Could you check a few things on this model? Use its own coordinates, in mm. A direction names the side the tool comes from. Coordinates: 2 decimals unless noted, no trailing zeros. Write each loop counter-clockwise with the first axis right and the second up, starting at its lowest first coordinate (ties: lowest second). Pieces come first, ordered by that corner, then holes.
Solid Edge part; units mm, degrees
sketch "Sketch1" plane through (0, 0, 0) normal (0, -1, 0) x (1, 0, 0)
  arc A0 (150, -21) -> (158.7897, 19.072) centre (150, 0) ccw
  line L0 (158.7897, 19.072) -> (43.7897, 72.072)
  arc A1 (17.4762, 64.5723) -> (43.7897, 72.072) centre (35, 53) cw
  line L1 (-17.5238, 11.5723) -> (17.4762, 64.5723)
  arc A2 (-17.5238, 11.5723) -> (0, -21) centre (0, 0) ccw
  line L2 (150, -21) -> (0, -21)
  line L3 (14.2527, 66.7011) -> (-20.7473, 13.7011)
  arc A3 (-20.7473, 13.7011) -> (0, -24.8631) centre (0, 0) ccw
  line L4 (0, -24.8631) -> (150, -24.8631)
  arc A4 (163.0772, 21.3496) -> (150, -24.8631) centre (150, 0.0936) cw
  line L5 (163.0772, 21.3496) -> (45.4066, 75.5804)
  arc A5 (14.2527, 66.7011) -> (45.4066, 75.5804) centre (35, 53) cw
extrude "Protrusion1" add sketch "Sketch1" along normal mid plane 34
properties material "ABS Plastic, medium impact"
1. Please list where these lines run through material, in increasing order: line 1 along Z through (x, y) = (45, 4); line 2 along X through (y, z) = (9, 15); line 3 along Z through (x, y) = (32, -14).
Verdict:
line 1: z = -24.86 to -21, 71.51 to 75.76
line 2: x = -19.89 to -15.26, 164.7 to 170.02
line 3: z = -24.86 to -21, 73.78 to 77.68
2. For pin 1 (2 mm diameter, centred on y = -2.5, z = 23.5, fed in from +X); pin 2 (6 mm diameter, centred on y = -7.5, z = -7, fed in from +X); pin 3 (6 mm diameter, centred on y = 3.5, z = 4.5, fed in from -X), each with a flat end and sliding along its axis, tell me the tip position at first contact or that it passes through.
Verdict:
pin 1: stops at x = 160.58
pin 2: stops at x = 174.62
pin 3: stops at x = -24.82
3. I want a section at C-C on x = 92. Please give me the cut outline in (y, z).
Verdict:
outline: (-17, -24.86) - (17, -24.86) - (17, -21) - (-17, -21) - close; (-17, 49.85) - (17, 49.85) - (17, 54.11) - (-17, 54.11) - close
4. If we mould it in two halves opening along X, with no side actions, what happens to faces 1 (the face through (-0.27, 0.24, 37.7)), 2 (the face through (27.948, 0.238, 76.842)), 3 (the face through (74, 0, -24.863)), 4 (the face through (29.044, 0.238, 73.138))? For each: pulls with the +X half, pulls with the -X half, needs draft (parallel to the pull), parting line crosses it, or undercut.
Verdict:
face 1: undercut
face 2: parting line crosses it
face 3: needs draft
face 4: undercut
5. I want a section at B-B on z = 42. Please give me the cut outline in (x, y).
Verdict:
outline: (-2.06, -17) - (2.57, -17) - (2.57, 17) - (-2.06, 17) - close; (109.04, -17) - (118.27, -17) - (118.27, 17) - (109.04, 17) - close
6. I want a section at A-A on y = -8. Please give me the cut outline in (x, z), plus the area to 3 significant figures.
Verdict:
outline: (-20.75, 13.7) arc R24.86 ccw to (0, -24.86) - (150, -24.86) arc R24.96 ccw to (163.08, 21.35) - (45.41, 75.58) arc R24.86 ccw to (14.25, 66.7) - close; hole (-17.52, 11.57) arc R21 ccw to (0, -21) - (150, -21) arc R21 ccw to (158.79, 19.07) - (43.79, 72.07) arc R21 ccw to (17.48, 64.57) - close
area: 1,880 mm2
7. On a 3-axis mill with a long thin cutter (end or side, diameter ignored), from which of +Z, -Z, +X, -X, +Y, -Y can I reach the whole of each face in a straight line? I mean faces 5 (the face through (105.066, 0.238, 48.085)), 6 (the face through (170.594, 0.238, -4.109)). Say none if no direction works.
Verdict:
face 5: +Z, +X, +Y, -Y
face 6: +Y, -Y
